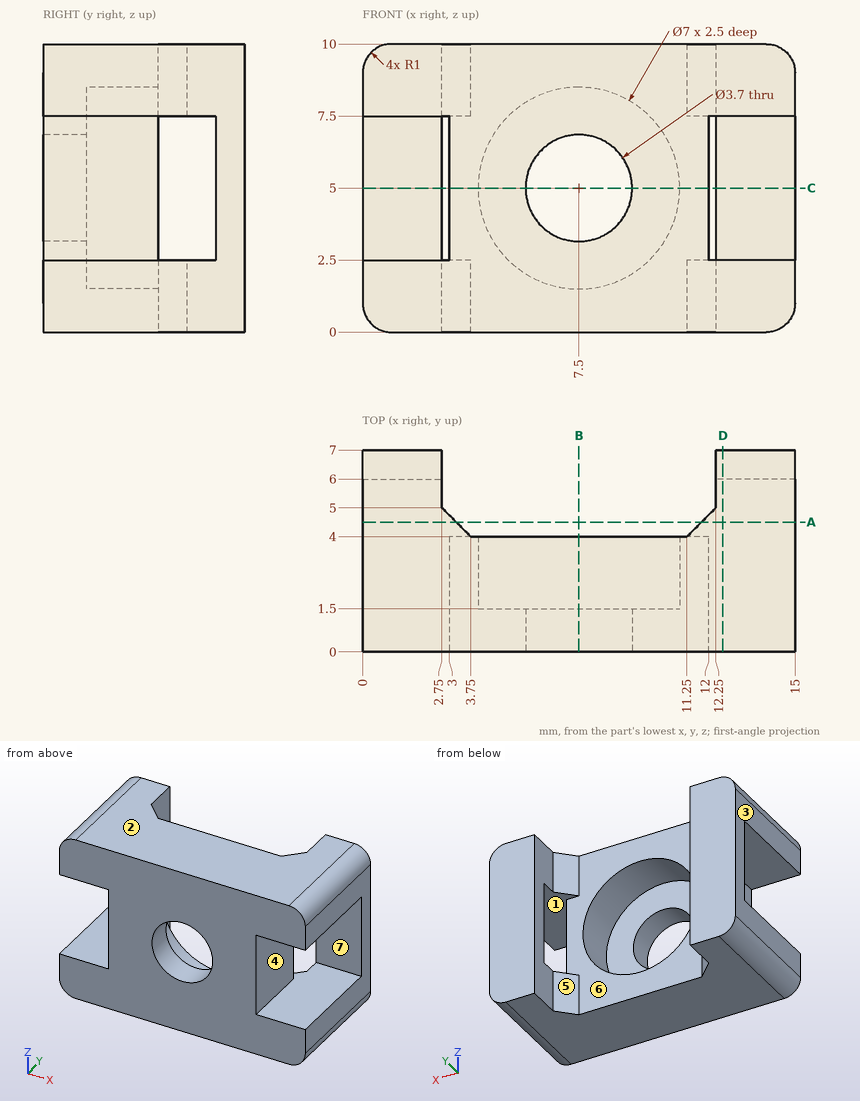
Design review of the part shown in the three views and the two pictorial views. Dimensions are in mm from the part's minimum x, y and z. A direction names the side the tool comes from. Give positions to 0.01 mm unless a question says otherwise; leave off trailing zeros. Loops run counter-clockwise (first coordinate to the right, second up) from the corner with the lowest first, then second, coordinate; pieces in that order, holes last. Notation, with made-up numbers: (13, 31.25) -> (28, 31.25) arc R24 cw to (28, 67.25) -> close; hole circle Ø6 at (14, 18). An arc over 180 degrees is marked (long way). Write each question's results on one line, items separated by ' | '.
1) Take a section at C-C, the plane z = 5. Give the boundary of the cut face in (x, y).
Conclusion:
outline: (0, 6) -> (2.75, 6) -> (2.75, 7) -> (0, 7) -> close; (3, 0) -> (5.65, 0) -> (5.65, 1.5) -> (4, 1.5) -> (4, 4) -> (3, 4) -> close; (9.35, 0) -> (12, 0) -> (12, 4) -> (11, 4) -> (11, 1.5) -> (9.35, 1.5) -> close; (12.25, 6) -> (15, 6) -> (15, 7) -> (12.25, 7) -> close
2) Tool access review of the marked faces 4, 5, 6 and 7: name each direction out of +Z, -Z, +X, -X, +Y, -Y from which nothing blocks a thin tool from reaching the whole face with its end or side.
Conclusion:
face 4: +X, +Y, -Y | face 5: +Z, -Z, +Y | face 6: +Y | face 7: +X, -X, -Y
3) Take a section at A-A, the plane y = 4.5. Give the boundary of the cut face in (x, z), plus the area to 3 significant figures.
Conclusion:
outline: (0, 1) arc R1 ccw to (1, 0) -> (3.25, 0) -> (3.25, 2.5) -> (0, 2.5) -> close; (0, 7.5) -> (3.25, 7.5) -> (3.25, 10) -> (1, 10) arc R1 ccw to (0, 9) -> close; (11.75, 0) -> (14, 0) arc R1 ccw to (15, 1) -> (15, 2.5) -> (11.75, 2.5) -> close; (11.75, 7.5) -> (15, 7.5) -> (15, 9) arc R1 ccw to (14, 10) -> (11.75, 10) -> close | area: 31.6 mm^2
4) Draft analysis for pull direction Z (two halves, no side actions). For the marked faces 1, 2 and 3, state which applies: pulls with the +Z half, pulls with the -Z half, needs draft (parallel to the pull), parting line crosses it, or undercut.
Conclusion:
face 1: undercut | face 2: pulls with the +Z half | face 3: needs draft
5) Take a section at B-B, the plane x = 7.5. Give the boundary of the cut face in (y, z), plus the area to 4 significant figures.
Conclusion:
outline: (0, 0) -> (4, 0) -> (4, 1.5) -> (1.5, 1.5) -> (1.5, 3.15) -> (0, 3.15) -> close; (0, 6.85) -> (1.5, 6.85) -> (1.5, 8.5) -> (4, 8.5) -> (4, 10) -> (0, 10) -> close | area: 16.95 mm^2
6) Take a section at D-D, the plane x = 12.5. Give the boundary of the cut face in (y, z), plus the area to 3 significant figures.
Conclusion:
outline: (0, 0) -> (7, 0) -> (7, 10) -> (0, 10) -> (0, 7.5) -> (6, 7.5) -> (6, 2.5) -> (0, 2.5) -> close | area: 40.0 mm^2
7) Insertion check: pin 1 Ø3 at (x, y) = (1.5, 2) entering from -Z; pin 2 Ø2.5 at (x, z) = (5.5, 6.5) entering from +Y; pin 3 Ø5.5 at (x, z) = (7.5, 4.5) entering from +Y; pin 4 Ø3 at (x, z) = (1, 5.5) entering from -Y. Each pin has a flat end and moves straight along its axis. Give the tip position at first contact, or say it passes through.
Conclusion:
pin 1: stops at z = 0 | pin 2: stops at y = 4 | pin 3: stops at y = 1.5 | pin 4: stops at y = 6
8) For line 1 along X through (y, z) = (6.5, 2.75); line 2 along Z through (x, y) = (7.5, 2.75); line 3 along Z through (x, y) = (13.25, 5.75), list the stretches that pass through material, from the lowest coordinate up. Write a range as from..to.
Conclusion:
line 1: x = 0..2.75, 12.25..15 | line 2: z = 0..1.5, 8.5..10 | line 3: z = 0..2.5, 7.5..10
